Could you check a few things on this model? Use its own coordinates, in mm. Face numbers are marked on the shaded views. A direction names the side the tool comes from. Coordinates: 2 decimals unless noted, no trailing zeros. Order: outer loops, then holes, each group sorted by start corner. A loop starts at its lowest first (then second) coordinate and runs counter-clockwise, first axis right, second up. Notation, with made-up numbers: (10, 66.5) -> (20, 66.5) arc R13 cw to (20, 70.5) -> close; hole circle Ø10 at (-13.5, 81). An arc over 180 degrees is marked (long way). Put each result on its own line as item: value. Start each with the question number.
Q1. For the marked faces 1 and 2, which set-ups out of +Z, -Z, +X, -X, +Y, -Y let a thin tool reach every point of the face, with its end or its side?
Q2. If we section it at B-B (x = 9.75): Please give me the cut outline in (y, z).
Q3. Will these pins go through, and if not, where does the flat tip stop? pin 1 (8 mm diameter, centred on x = 10.5, z = -3.5, fed in from -Y); pin 2 (8 mm diameter, centred on x = -1.5, y = 2, fed in from -Z); pin 3 (1.2 mm diameter, centred on y = 0, z = 1.5, fed in from +X); pin 4 (0.8 mm diameter, centred on y = 1.5, z = 2, fed in from -X).
Q4. If we section it at A-A (y = 2): Please give me the cut outline in (x, z).
Q5. If we section it at C-C (y = -9.5): Please give me the cut outline in (x, z), and give its area (3 significant figures).
Q6. Please list where these lines run through material, in increasing order: line 1 along Z through (x, y) = (-1, 12.5); line 2 along X through (y, z) = (-10, -9); line 3 along X through (y, z) = (-3, -14).
Q7. We'd pull the mould along Z, two halves only. Please class the marked faces 3, 4, 5 and 6: +Z half, -Z half, draft (parallel to the pull), parting line (faces both ways), or undercut.
Q8. If we section it at D-D (x = 3): Please give me the cut outline in (y, z), and give its area (4 significant figures).
from build123d import *

# Parameters (mm, degrees)
SKETCH_1_W          = 35
SKETCH_1_H          = 32.5
EXTRUDE_1_DEPTH     = 2.5
EXTRUDE_2_DEPTH     = 32.5
FILLET_1_R          = 2
FILLET_2_R          = 5
SKETCH_3_R          = 1.5
CUT_EXTRUDE_1_DEPTH = 10
CUT_EXTRUDE_2_DEPTH = 10


with BuildPart() as part:
    # 草图1 → 凸台-拉伸1 (new body)
    with BuildSketch(Plane.XY):
        Rectangle(SKETCH_1_W, SKETCH_1_H)
    extrude(amount=EXTRUDE_1_DEPTH)

    # 草图2 → 凸台-拉伸2 (add)
    with BuildSketch(Plane.XZ.offset(16.25)):
        Polygon((-13.675929559, -24.871935947), (-14.98280876, 0.054942395), (-17.43216424, 0.054942395), (-16.118570831, -25), align=None)
        Polygon((16.118570831, -27.5), (13.675929559, -27.371935947), (15.108562872, 0.305766553), (17.5, 0.82312635), align=None)
    extrude(amount=-EXTRUDE_2_DEPTH)

    # 圆角1
    fillet_1_edges = [part.edges().sort_by_distance(p)[0] for p in [
        (17.5, 0, 2.5),
        (-14.979928212, 0, 0),
        (15.092736004, 0, 0),
        (-17.5, 0, 2.5),
    ]]
    fillet(fillet_1_edges, radius=FILLET_1_R)

    # 圆角2
    fillet_2_edges = [part.edges().sort_by_distance(p)[0] for p in [
        (-14.897250195, -16.25, -24.935967973),
        (-14.897250195, 16.25, -24.935967973),
        (14.897250195, -16.25, -27.435967973),
        (14.897250195, 16.25, -27.435967973),
    ]]
    fillet(fillet_2_edges, radius=FILLET_2_R)

    # 草图3 → 切除-拉伸1 (cut)
    with BuildSketch(Plane(origin=(17.418416378, 0, -0.849563998), x_dir=(-0.048715984, 0, -0.998812672), z_dir=(0.998812672, 0, -0.048715984))):
        with Locations((22.256634944, 0)):
            Circle(SKETCH_3_R)
    extrude(amount=-CUT_EXTRUDE_1_DEPTH, mode=Mode.SUBTRACT)

    # 草图4 → 切除-拉伸2 (cut)
    with BuildSketch(Plane.XY.offset(2.5)):
        with BuildLine():
            Line((12.5, 2.75), (12.5, -2.75))
            ThreePointArc((12.5, -2.75), (9.75, -5.5), (7, -2.75))
            Line((7, -2.75), (7, 2.75))
            ThreePointArc((7, 2.75), (9.75, 5.5), (12.5, 2.75))
        make_face()
    extrude(amount=-CUT_EXTRUDE_2_DEPTH, mode=Mode.SUBTRACT)


solid = part.part
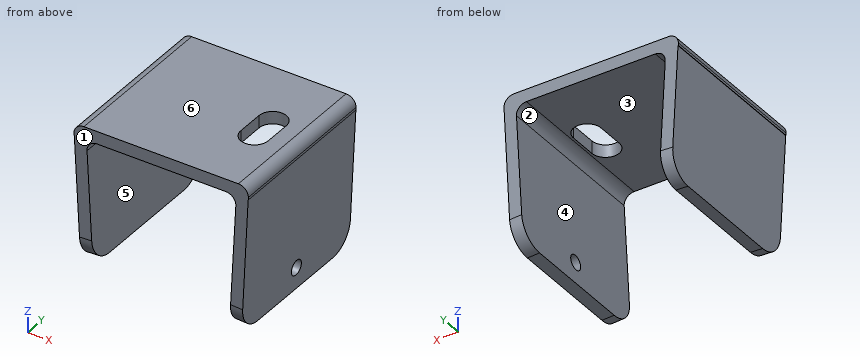
The answers:
1. face 1: +Z, -Z, +X, -X, -Y
1. face 2: +Y, -Y
2. outline: (-16.25, 0) -> (-5.5, 0) -> (-5.5, 2.5) -> (-16.25, 2.5) -> close; (5.5, 0) -> (16.25, 0) -> (16.25, 2.5) -> (5.5, 2.5) -> close
3. pin 1: y = -16.25
3. pin 2: z = 0
3. pin 3: x = 17.46
3. pin 4: x = -17.17
4. outline: (-17.5, 0) -> (-17.43, 0) -> (-16.12, -25) -> (-13.68, -24.87) -> (-14.87, -2.1) arc R2 cw to (-12.87, 0) -> (7, 0) -> (7, 2.5) -> (-15.5, 2.5) arc R2 ccw to (-17.5, 0.5) -> close; (12.5, 0) -> (12.99, 0) arc R2 cw to (14.98, -2.1) -> (13.68, -27.37) -> (16.12, -27.5) -> (17.46, 0) -> (17.5, 0) -> (17.5, 0.5) arc R2 ccw to (15.5, 2.5) -> (12.5, 2.5) -> close
5. outline: (-17.5, 0) -> (-17.43, 0) -> (-16.12, -25) -> (-13.68, -24.87) -> (-14.87, -2.1) arc R2 cw to (-12.87, 0) -> (12.99, 0) arc R2 cw to (14.98, -2.1) -> (13.68, -27.37) -> (16.12, -27.5) -> (17.46, 0) -> (17.5, 0) -> (17.5, 0.5) arc R2 ccw to (15.5, 2.5) -> (-15.5, 2.5) arc R2 ccw to (-17.5, 0.5) -> close
5. area: 215 mm^2
6. line 1: 0 to 2.5
6. line 2: -16.96 to -14.51, 14.63 to 17.02
6. line 3: -16.7 to -14.25, 14.37 to 16.78
7. face 3: -Z half
7. face 4: undercut
7. face 5: undercut
7. face 6: +Z half
8. outline: (-16.25, 0) -> (16.25, 0) -> (16.25, 2.5) -> (-16.25, 2.5) -> close
8. area: 81.25 mm^2
